Here's how the part is built. I have some questions about the finished solid (model axes, mm). Face numbers are marked on the shaded views. A direction names the side the tool comes from. Round coordinates to 2 decimals unless told otherwise and drop trailing zeros. Write each loop counter-clockwise with the first axis right and the second up, starting at its lowest first coordinate (ties: lowest second). Pieces come first, ordered by that corner, then holes. Notation, with made-up numbers: M 40.25,62.25 L 64.25,62.25 A17 cw 64.25,95.25 Z; hole C -4.75,60 d4. An arc over 180 degrees is marked long. Use one line per item in the form item = value. Start each with the question number.
Q1. I'm going to push flat-ended pins straight in: pin 1 Ø0.9 at (x, z) = (0.5, 2.5) entering from +Y; pin 2 Ø0.8 at (x, y) = (-3.5, 10) entering from +Z; pin 3 Ø0.6 at (x, y) = (3.5, 9.5) entering from -Z. Where does each tip first touch, or does it pass through?
Q2. I want a section at B-B on y = 9.75. List the corners of the cut face in (x, z) for me.
Q3. I want a section at D-D on y = 3.15. List the corners of the cut face in (x, z) for me, and give its area (3 significant figures).
Q4. I want a section at A-A on x = 0. List the corners of the cut face in (y, z) for me.
Q5. For the marked faces 1 and 2, which set-ups out of +Z, -Z, +X, -X, +Y, -Y let a thin tool reach every point of the face, with its end or its side?
Q6. I want a section at C-C on z = 1. State how many separate pieces and enclosed holes the cut face has, and give its area (3 significant figures).
Q7. We'd pull the mould along Z, two halves only. Please class the marked faces 3, 4 and 5: +Z half, -Z half, draft (parallel to the pull), parting line (faces both ways), or undercut.
Q8. I need wall thicknesses on line 1 along X through (y, z) = (1.5, 2); line 2 along Y through (x, z) = (3.8, 0); line 3 along X through (y, z) = (2.15, 0). Which ranges of each line are inside material? Lowest first, please. Write a range as from..to.
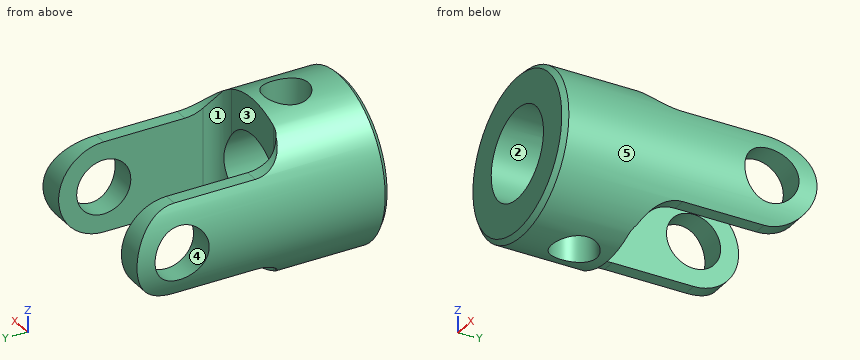
```python
from build123d import *

# Parameters (mm, degrees)
SKETCH1_R               = 4.5
SKETCH1_R_2             = 2.5
BOSS_EXTRUDE1_DEPTH     = 14
CUT_EXTRUDE1_DEPTH      = 16.378556499
CUT_EXTRUDE1_DEPTH_BACK = 16.378556499
SKETCH2_R               = 1.25
CUT_EXTRUDE2_DEPTH      = 16.378556652
CUT_EXTRUDE2_DEPTH_BACK = 16.378556652
SKETCH3_R               = 1.5
CHAMFER1_SIZE           = 0.25


with BuildPart() as part:
    # Sketch1 → Boss-Extrude1 (new body)
    with BuildSketch(Plane(origin=(0, 0, 0), x_dir=(1, 0, 0), z_dir=(0, 1, 0))):
        with Locations(Location((0, 0, 0), (0, 0, 270))):
            Circle(SKETCH1_R)
        with Locations(Location((0, 0, 0), (0, 0, 270))):
            Circle(SKETCH1_R_2, mode=Mode.SUBTRACT)
    extrude(amount=BOSS_EXTRUDE1_DEPTH)

    # Sketch2 → Cut-Extrude1 (cut, two sides: drawn at the far end of the back side and taken through both)
    with BuildSketch(Plane.XY.offset(-CUT_EXTRUDE1_DEPTH_BACK)):
        with Locations((0, 3.15)):
            Circle(SKETCH2_R)
        with BuildLine():
            Line((-3, 14), (3, 14))
            Line((3, 14), (3, 6))
            ThreePointArc((3, 6), (2.707106781, 5.292893219), (2, 5))
            Line((2, 5), (-2, 5))
            ThreePointArc((-2, 5), (-2.707106781, 5.292893219), (-3, 6))
            Line((-3, 6), (-3, 14))
        make_face()
    extrude(amount=CUT_EXTRUDE1_DEPTH + CUT_EXTRUDE1_DEPTH_BACK, mode=Mode.SUBTRACT)

    # Sketch3 → Cut-Extrude2 (cut, two sides: drawn at the far end of the back side and taken through both)
    with BuildSketch(Plane(origin=(0, 0, 0), x_dir=(0, 0, -1), z_dir=(1, 0, 0)).offset(-CUT_EXTRUDE2_DEPTH_BACK)):
        with Locations((0, 11.5)):
            Circle(SKETCH3_R)
        with BuildLine():
            Line((2.5, 11.5), (2.5, 7))
            ThreePointArc((2.5, 7), (3.085786438, 5.585786438), (4.5, 5))
            Line((4.5, 5), (4.5, 15))
            Line((4.5, 15), (-4.5, 15))
            Line((-4.5, 15), (-4.5, 5))
            ThreePointArc((-4.5, 5), (-3.085786438, 5.585786438), (-2.5, 7))
            Line((-2.5, 7), (-2.5, 11.5))
            ThreePointArc((-2.5, 11.5), (0, 14), (2.5, 11.5))
        make_face()
    extrude(amount=CUT_EXTRUDE2_DEPTH + CUT_EXTRUDE2_DEPTH_BACK, mode=Mode.SUBTRACT)

    # Chamfer1
    chamfer1_edges = [part.edges().sort_by_distance(p)[0] for p in [
        (0, 0, -4.5),
    ]]
    chamfer(chamfer1_edges, length=CHAMFER1_SIZE)


solid = part.part
```
Reported:
q1.pin_1 = 5
q1.pin_2 = 2.5
q1.pin_3 = -2.5
q2.outline = M -3.74,-2.5 L -3,-2.5 L -3,2.5 L -3.74,2.5 A4.5 ccw Z; M 3,-2.5 L 3.74,-2.5 A4.5 ccw 3.74,2.5 L 3,2.5 Z
q3.outline = M -1.25,-4.32 L -1.25,-2.17 A2.5 cw -1.25,2.17 L -1.25,4.32 A4.5 ccw Z; M 1.25,-4.32 A4.5 ccw 1.25,4.32 L 1.25,2.17 A2.5 cw 1.25,-2.17 Z
q3.area = 33.7 mm^2
q4.outline = M 0,-4.25 L 0.25,-4.5 L 1.9,-4.5 L 1.9,-2.5 L 0,-2.5 Z; M 0,2.5 L 1.9,2.5 L 1.9,4.5 L 0.25,4.5 L 0,4.25 Z; M 4.4,-4.5 L 5,-4.5 L 5,-2.5 L 4.4,-2.5 Z; M 4.4,2.5 L 5,2.5 L 5,4.5 L 4.4,4.5 Z
q5.face_1 = +Z, -Z, +Y
q5.face_2 = +Y, -Y
q6.separate_pieces = 4
q6.enclosed_holes = 0
q6.area = 39.5 mm^2
q7.face_3 = draft
q7.face_4 = undercut
q7.face_5 = parting line
q8.line_1 = -4.03..-1.5, 1.5..4.03
q8.line_2 = 0..10, 13..14
q8.line_3 = -4.5..-2.5, 2.5..4.5
